```python
from build123d import *

# Parameters (mm, degrees)
SKETCH_1_R          = 17.5
EXTRUDE_1_DEPTH     = 5
SKETCH_10_W         = 76
SKETCH_10_H         = 40
SKETCH_10_R         = 2.75
EXTRUDE_2_DEPTH     = 5
SKETCH_11_R         = 27.5
SKETCH_11_R_2       = 17.5
EXTRUDE_3_DEPTH     = 10
SKETCH_12_R         = 2.25
CUT_EXTRUDE_6_DEPTH = 40


with BuildPart() as part:
    # 草图1 → 凸台-拉伸1 (new body)
    with BuildSketch(Plane.XY):
        with BuildLine():
            Line((-48, 109.07), (-48, 0))
            Line((-48, 0), (48, 0))
            Line((48, 0), (48, 109.07))
            ThreePointArc((48, 109.07), (0, 145.07), (-48, 109.07))
        make_face()
        with Locations((0, 95.07)):
            Circle(SKETCH_1_R, mode=Mode.SUBTRACT)
    extrude(amount=EXTRUDE_1_DEPTH)

    # 草图10 → 凸台-拉伸2 (add)
    with BuildSketch(Plane.XY.offset(5)):
        with Locations((0, -20)):
            Rectangle(SKETCH_10_W, SKETCH_10_H)
        with Locations((25, -20)):
            Circle(SKETCH_10_R, mode=Mode.SUBTRACT)
        with Locations((-25, -20)):
            Circle(SKETCH_10_R, mode=Mode.SUBTRACT)
        with Locations((0, -20)):
            Circle(SKETCH_10_R, mode=Mode.SUBTRACT)
    extrude(amount=-EXTRUDE_2_DEPTH)

    # 草图11 → 凸台-拉伸3 (add)
    with BuildSketch(Plane.XY.offset(5)):
        with Locations((0, 95.07)):
            Circle(SKETCH_11_R)
        with Locations((0, 95.07)):
            Circle(SKETCH_11_R_2, mode=Mode.SUBTRACT)
    extrude(amount=EXTRUDE_3_DEPTH)

    # 草图12 → 切除-拉伸6 (cut)
    with BuildSketch(Plane.XY.offset(15)):
        with Locations((0, 117.57)):
            Circle(SKETCH_12_R)
        with Locations((15.909902577, 110.979902577)):
            Circle(SKETCH_12_R)
        with Locations((22.5, 95.07)):
            Circle(SKETCH_12_R)
        with Locations((15.909902577, 79.160097423)):
            Circle(SKETCH_12_R)
        with Locations((0, 72.57)):
            Circle(SKETCH_12_R)
        with Locations((-15.909902577, 79.160097423)):
            Circle(SKETCH_12_R)
        with Locations((-22.5, 95.07)):
            Circle(SKETCH_12_R)
        with Locations((-15.909902577, 110.979902577)):
            Circle(SKETCH_12_R)
    extrude(amount=-CUT_EXTRUDE_6_DEPTH, mode=Mode.SUBTRACT)


solid = part.part
```
Input: part model. Units: mm. Frame: model coordinates. A direction names the side the tool comes from. Round coordinates to 2 decimals unless told otherwise and drop trailing zeros. Order: outer loops, then holes, each group sorted by start corner. A loop starts at its lowest first (then second) coordinate and runs counter-clockwise, first axis right, second up. Notation, with made-up numbers: (43, 37) - (102, 37) arc R21 ccw to (102, 55) - close; hole circle Ø8 at (86, 48.25). An arc over 180 degrees is marked (long way). Answer in a Markdown table with one row per item.
Item 1: Pin query (flat end, axial travel): pin 1 (7 mm diameter, centred on x = -25, y = -20, fed in from +Z); pin 2 (21 mm diameter, centred on x = 0, y = 95.07, fed in from -Z); pin 3 (7 mm diameter, centred on x = 15.91, y = 79.16, fed in from +Z); pin 4 (1.5 mm diameter, centred on y = -22, z = 3.5, fed in from +X). Return the tip coordinate at first contact, or that it passes through.
Model answer:
| item | result |
|---|---|
| pin 1 | stops at z = 5 |
| pin 2 | passes through |
| pin 3 | stops at z = 15 |
| pin 4 | stops at x = 38 |
Item 2: Mould query, pull axis Y, two halves, no side actions, for faces 1 (the flat face through (-1, -40, 3)), 2 (the cylindrical face through (-27.747, -19.879, 2.535)), 3 (the flat face through (-48, 55, 2)). Classes: released by +Y, released by -Y, zero draft, split by the parting line, or undercut.
Model answer:
| item | result |
|---|---|
| face 1 | released by -Y |
| face 2 | undercut |
| face 3 | zero draft |
Item 3: Reachability of faces 4 (the cylindrical face through (-16.2, 113.21, 7.6)), 5 (the cylindrical face through (12.69, 70.673, 9.93)), 6 (the flat face through (43, 0, 2)) from +Z, -Z, +X, -X, +Y, -Y: full face, straight path, thin tool, end or side. Return the list, or none.
Model answer:
| item | result |
|---|---|
| face 4 | +Z, -Z |
| face 5 | +Z |
| face 6 | +Z, -Z, +X, -Y |
Item 4: Section query B-B (y = -20). Return the cut outline in (x, z).
Model answer:
| item | result |
|---|---|
| outline | (-38, 0) - (-27.75, 0) - (-27.75, 5) - (-38, 5) - close; (-22.25, 0) - (-2.75, 0) - (-2.75, 5) - (-22.25, 5) - close; (2.75, 0) - (22.25, 0) - (22.25, 5) - (2.75, 5) - close; (27.75, 0) - (38, 0) - (38, 5) - (27.75, 5) - close |
Item 5: Section query A-A (x = 0). Return the cut outline in (y, z), then the cut area to 3 significant figures.
Model answer:
| item | result |
|---|---|
| outline | (-40, 0) - (-22.75, 0) - (-22.75, 5) - (-40, 5) - close; (-17.25, 0) - (70.32, 0) - (70.32, 15) - (67.57, 15) - (67.57, 5) - (-17.25, 5) - close; (74.82, 0) - (77.57, 0) - (77.57, 15) - (74.82, 15) - close; (112.57, 0) - (115.32, 0) - (115.32, 15) - (112.57, 15) - close; (119.82, 0) - (145.07, 0) - (145.07, 5) - (122.57, 5) - (122.57, 15) - (119.82, 15) - close |
| area | 788 mm² |
Item 6: Section query D-D (z = 2.75). Give the number of separate pieces and of enclosed holes in the cut face, then the cut area to 3 significant figures.
Model answer:
| item | result |
|---|---|
| separate pieces | 1 |
| enclosed holes | 12 |
| area | 14,900 mm² |
Item 7: Section query C-C (x = 10). Return the cut outline in (y, z).
Model answer:
| item | result |
|---|---|
| outline | (-40, 0) - (80.71, 0) - (80.71, 15) - (69.45, 15) - (69.45, 5) - (-40, 5) - close; (109.43, 0) - (144.06, 0) - (144.06, 5) - (120.69, 5) - (120.69, 15) - (109.43, 15) - close |
Item 8: Line query: line 1 (Y direction, x = 0, z = 9.25); line 2 (Y direction, x = 0, z = 4); line 3 (Y direction, x = 14, z = 6.75). Output: solid intervals per line, ascending.
Model answer:
| item | result |
|---|---|
| line 1 | y = 67.57 to 70.32, 74.82 to 77.57, 112.57 to 115.32, 119.82 to 122.57 |
| line 2 | y = -40 to -22.75, -17.25 to 70.32, 74.82 to 77.57, 112.57 to 115.32, 119.82 to 145.07 |
| line 3 | y = 71.4 to 77.97, 80.35 to 84.57, 105.57 to 109.79, 112.17 to 118.74 |
